from build123d import *

# Parameters (mm, degrees)
SKETCH1_R           = 27
BOSS_EXTRUDE1_DEPTH = 10
FILLET1_R           = 5
SKETCH2_R           = 5
CUT_EXTRUDE1_DEPTH  = 10


with BuildPart() as part:
    # Sketch1 → Boss-Extrude1 (new body)
    with BuildSketch(Plane(origin=(0, 0, 0), x_dir=(1, 0, 0), z_dir=(0, 1, 0))):
        Circle(SKETCH1_R)
    extrude(amount=BOSS_EXTRUDE1_DEPTH)

    # Fillet1
    fillet1_edges = [part.edges().sort_by_distance(p)[0] for p in [
        (-27, 10, 0),
    ]]
    fillet(fillet1_edges, radius=FILLET1_R)

    # Sketch2 → Cut-Extrude1 (cut)
    with BuildSketch(Plane(origin=(0, 10, 0), x_dir=(1, 0, 0), z_dir=(0, 1, 0))):
        with Locations((11.112679592, -8.515183631)):
            Circle(SKETCH2_R)
    extrude(amount=-CUT_EXTRUDE1_DEPTH, mode=Mode.SUBTRACT)


solid = part.part
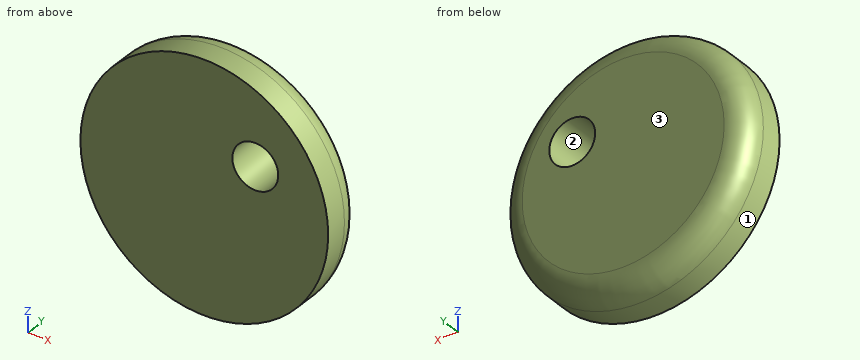
Verification items for the finished model (mm, model axes). Face numbers are marked on the shaded views. Round coordinates to 2 decimals unless told otherwise and drop trailing zeros. Order: outer loops, then holes, each group sorted by start corner. A loop starts at its lowest first (then second) coordinate and runs counter-clockwise, first axis right, second up.
1. Release check for a two-part mould opening along X. For the marked faces 1, 2 and 3 record: +X half, -X half, draft (parallel to the pull), parting line (faces both ways), or undercut.
Final values:
face 1: parting line
face 2: undercut
face 3: draft
2. Section check B-B on z = 0. Record the cut outline in (x, y), then the cut area to 3 significant figures.
Final values:
outline: (-27, 0) - (27, 0) - (27, 5) arc R5 ccw to (22, 10) - (-22, 10) arc R5 ccw to (-27, 5) - close
area: 529 mm2
3. Section check D-D on y = 8. Record the cut outline in (x, z).
Final values:
outline: circle Ø52 at (0, 0); hole circle Ø10 at (11.11, 8.52)
4. Section check C-C on y = 3.5. Record the cut outline in (x, z).
Final values:
outline: circle Ø54 at (0, 0); hole circle Ø10 at (11.11, 8.52)
5. Go/stop test with flat-tipped pins: P1, Ø1, axis at x = -7, y = 4.5, coming from the +Z side; P2, Ø2, axis at y = 6, z = -14.5, coming from the +X side; P3, Ø4, axis at x = -12, y = 7, coming from the +Z side. Record where each tip stops, or that it passes through.
Final values:
P1: stops at z = 26.21
P2: stops at x = 23.3
P3: stops at z = 24.86
6. Thickness scan on L1, parallel to Y at x = 20, z = 9.5; L2, parallel to X at y = 8.75, z = -12.5; L3, parallel to Z at x = 14, y = 7. Record the ranges inside material, lowest first.
Final values:
L1: y = 0 to 10
L2: x = -22 to 22
L3: z = -22.6 to 4.43, 12.6 to 22.6
7. Section check A-A on x = 0. Record the cut outline in (y, z).
Final values:
outline: (0, -27) - (5, -27) arc R5 ccw to (10, -22) - (10, 22) arc R5 ccw to (5, 27) - (0, 27) - close
